Design review of the part built by this model. Coordinates are the model's own, in mm. Give positions to 0.01 mm unless a question says otherwise; leave off trailing zeros. Loops run counter-clockwise (first coordinate to the right, second up) from the corner with the lowest first, then second, coordinate; pieces in that order, holes last. Notation, with made-up numbers: (80.25, 21.5) -> (100.25, 21.5) arc R27 cw to (100.25, 57.5) -> close; hole circle Ø8 at (39, 9). An arc over 180 degrees is marked (long way). Answer as CSV lines item,"result".
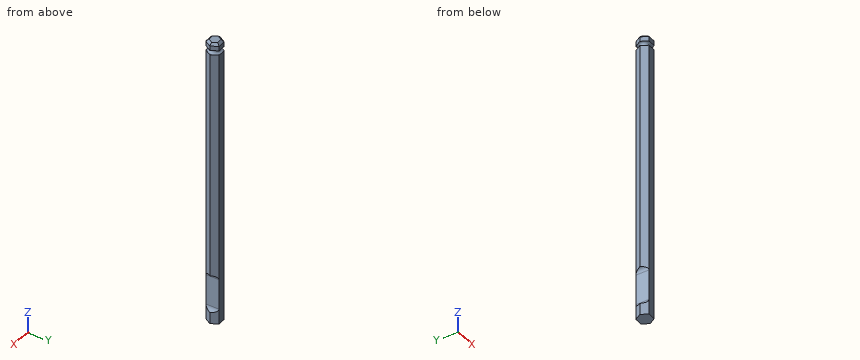
from build123d import *

# Parameters (mm, degrees)
SALIENTE_EXTRUIR1_DEPTH    = 95
CHAFL_N1_SIZE              = 0.75
CROQUIS2_R                 = 0.75
CORTAR_EXTRUIR1_DEPTH      = 96.057548464
CORTAR_EXTRUIR1_DEPTH_BACK = 96.057548464


with BuildPart() as part:
    # Croquis1 → Saliente-Extruir1 (new body)
    with BuildSketch(Plane.XY):
        Polygon((1.25, -2.165063509), (2.5, 0), (1.25, 2.165063509), (-1.25, 2.165063509), (-2.5, 0), (-1.25, -2.165063509), align=None)
    extrude(amount=-SALIENTE_EXTRUIR1_DEPTH)

    # Chaflán1
    chafl_n1_edges = [part.edges().sort_by_distance(p)[0] for p in [
        (-1.875, -1.082531755, 0),
        (-1.875, 1.082531755, 0),
        (0, 2.165063509, 0),
        (1.875, 1.082531755, 0),
        (1.875, -1.082531755, 0),
        (0, -2.165063509, 0),
    ]]
    chamfer(chafl_n1_edges, length=CHAFL_N1_SIZE)

    # Croquis2 → Cortar-Revolución1 (revolve, cut)
    with BuildSketch(Plane(origin=(0, 0, 0), x_dir=(0, 0, -1), z_dir=(1, 0, 0)), mode=Mode.PRIVATE) as cortar_revoluci_n1_sk:
        with Locations((3, 2.165063509)):
            Circle(CROQUIS2_R)
    revolve(cortar_revoluci_n1_sk.sketch.rotate(Axis((0, 0, 0), (0, 0, 1)), 329.999999874), axis=Axis((0, 0, 0), (0, 0, 1)), mode=Mode.SUBTRACT)

    # Croquis5 → Cortar-Extruir1 (cut, two sides: drawn at the far end of the back side and taken through both)
    with BuildSketch(Plane(origin=(0, 0, 0), x_dir=(1, 0, 0), z_dir=(0, 1, 0)).offset(-CORTAR_EXTRUIR1_DEPTH_BACK)):
        with BuildLine():
            Line((-1.25, 90), (-1.25, 80))
            ThreePointArc((-1.25, 80), (-2.5, 78.75), (-3.75, 80))
            Line((-3.75, 80), (-3.75, 90))
            ThreePointArc((-3.75, 90), (-2.5, 91.25), (-1.25, 90))
        make_face()
        with BuildLine():
            Line((1.25, 90), (1.25, 80))
            ThreePointArc((1.25, 80), (2.5, 78.75), (3.75, 80))
            Line((3.75, 80), (3.75, 90))
            ThreePointArc((3.75, 90), (2.5, 91.25), (1.25, 90))
        make_face()
    extrude(amount=CORTAR_EXTRUIR1_DEPTH + CORTAR_EXTRUIR1_DEPTH_BACK, mode=Mode.SUBTRACT)


solid = part.part
Q1. We need section A-A, the plane z = -41. State the section outline as (x, y) points, and give its area (3 significant figures).
Filled sheet:
outline,"(-2.5, 0) -> (-1.25, -2.17) -> (1.25, -2.17) -> (2.5, 0) -> (1.25, 2.17) -> (-1.25, 2.17) -> close"
area,"16.2 mm^2"
Q2. Clearance check with a flat-ended pin moving along its axis: pin 1 Ø2 at (y, z) = (1.5, -59) entering from -X. State where the tip first meets the part, or that it passes through.
Filled sheet:
pin 1,"stops at x = -2.21"
Q3. To check wall thickness, follow probe 1 along Z at (x, y) = (1, -1.4); probe 2 along X at (y, z) = (-0.05, -81); probe 3 along X at (y, z) = (1.9, -27.5). State the ranges of each line that lie inside material, in increasing order. Write a range as from..to.
Filled sheet:
probe 1,"z = -95..-3.6, -2.4..-0.15"
probe 2,"x = -1.25..1.25"
probe 3,"x = -1.4..1.4"
